```python
from build123d import *

# Parameters (mm, degrees)
BOSS_EXTRUDE1_DEPTH             = 12.7
BOSS_EXTRUDE4_REACH             = 14.7
BOSS_EXTRUDE4_DIRECTION_2_REACH = 14.7
SKETCH6_W                       = 16.51
SKETCH6_H                       = 15.748
CUT_EXTRUDE2_DEPTH              = 46.72
SKETCH11_W                      = 15.24
SKETCH11_H                      = 7.62
CUT_EXTRUDE3_DEPTH              = 3.81
SKETCH15_R                      = 3.2385
CUT_EXTRUDE4_DEPTH              = 25.4
SKETCH16_W                      = 6.35
SKETCH16_H                      = 21.59
BOSS_EXTRUDE5_DEPTH             = 15.24
SKETCH17_R                      = 0.635
CUT_EXTRUDE5_DEPTH              = 26.4


with BuildPart() as part:
    # Sketch1 → Boss-Extrude1 (new body, symmetric)
    with BuildSketch(Plane.XY):
        with BuildLine():
            Line((-15.24, 16.002), (-15.24, -25.4))
            Line((-15.24, -25.4), (15.24, -25.4))
            Line((15.24, -25.4), (15.24, 16.002))
            Line((15.24, 16.002), (2.794, 16.002))
            Line((2.794, 16.002), (2.794, 28.3845))
            Line((2.794, 28.3845), (6.477, 28.3845))
            ThreePointArc((6.477, 28.3845), (6.946330803, 28.698096816), (6.836210245, 29.251710245))
            Line((6.836210245, 29.251710245), (3.452459265, 32.635461224))
            ThreePointArc((3.452459265, 32.635461224), (2.628423959, 33.186064013), (1.656408041, 33.37941))
            Line((1.656408041, 33.37941), (-1.656408041, 33.37941))
            ThreePointArc((-1.656408041, 33.37941), (-2.628423959, 33.186064013), (-3.452459265, 32.635461224))
            Line((-3.452459265, 32.635461224), (-6.836210245, 29.251710245))
            ThreePointArc((-6.836210245, 29.251710245), (-6.946330803, 28.698096816), (-6.477, 28.3845))
            Line((-6.477, 28.3845), (-2.794, 28.3845))
            Line((-2.794, 28.3845), (-2.794, 16.002))
            Line((-2.794, 16.002), (-15.24, 16.002))
        make_face()
        Polygon((-4.106115114, 7.112), (-8.212230229, 0), (-4.106115114, -7.112), (4.106115114, -7.112), (8.212230229, 0), (4.106115114, 7.112), align=None, mode=Mode.SUBTRACT)
    extrude(amount=BOSS_EXTRUDE1_DEPTH, both=True)

    # Boss-Extrude4: up to this face of the body (flat: up to its plane)
    boss_extrude4_end = Plane(part.part.faces().sort_by_distance((-6.334610257, 28.951479763, 12.7))[0])
    # Sketch10 → Boss-Extrude4 (add, up to the picked face)
    with BuildSketch(Plane.XY, mode=Mode.PRIVATE) as boss_extrude4_sk1:
        Polygon((-15.24, -25.4), (-15.24, -46.99), (-30.48, -46.99), (-30.48, -50.8), (-11.43, -50.8), (-11.43, -25.4), align=None)
    boss_extrude4_tool1 = split(extrude(boss_extrude4_sk1.sketch, amount=BOSS_EXTRUDE4_REACH, mode=Mode.PRIVATE), bisect_by=boss_extrude4_end, keep=Keep.BOTH, mode=Mode.PRIVATE)
    add(boss_extrude4_tool1.solids().sort_by_distance((-14.9225, -36.195, 0))[0])

    # Boss-Extrude4 direction 2: up to this face of the body (flat: up to its plane)
    boss_extrude4_direction_2_end = Plane(part.part.faces().sort_by_distance((-6.334610257, 28.951479763, -12.7))[0])
    # Sketch10 → Boss-Extrude4 direction 2 (add, up to the picked face)
    with BuildSketch(Plane.XY, mode=Mode.PRIVATE) as boss_extrude4_direction_2_sk1:
        Polygon((-15.24, -25.4), (-15.24, -46.99), (-30.48, -46.99), (-30.48, -50.8), (-11.43, -50.8), (-11.43, -25.4), align=None)
    boss_extrude4_direction_2_tool1 = split(extrude(boss_extrude4_direction_2_sk1.sketch, amount=-BOSS_EXTRUDE4_DIRECTION_2_REACH, mode=Mode.PRIVATE), bisect_by=boss_extrude4_direction_2_end, keep=Keep.BOTH, mode=Mode.PRIVATE)
    add(boss_extrude4_direction_2_tool1.solids().sort_by_distance((-14.9225, -36.195, 0))[0])

    # Sketch6 → Cut-Extrude2 (cut, through all)
    with BuildSketch(Plane(origin=(15.24, 0, 0), x_dir=(0, 0, -1), z_dir=(1, 0, 0))):
        with Locations((0, -17.526)):
            Rectangle(SKETCH6_W, SKETCH6_H)
    extrude(amount=-CUT_EXTRUDE2_DEPTH, mode=Mode.SUBTRACT)

    # Sketch11 → Cut-Extrude3 (cut)
    with BuildSketch(Plane(origin=(0, -46.99, 0), x_dir=(1, 0, 0), z_dir=(0, 1, 0))):
        with Locations((-22.86, 0)):
            Rectangle(SKETCH11_W, SKETCH11_H)
    extrude(amount=-CUT_EXTRUDE3_DEPTH, mode=Mode.SUBTRACT)

    # Sketch15 → Cut-Extrude4 (cut)
    with BuildSketch(Plane.XY.offset(12.7)):
        with Locations((0, -19.05)):
            Circle(SKETCH15_R)
    extrude(amount=-CUT_EXTRUDE4_DEPTH, mode=Mode.SUBTRACT)

    # Sketch16 → Boss-Extrude5 (add)
    with BuildSketch(Plane.ZY.offset(15.24)):
        with Locations((9.525, -36.195)):
            Rectangle(SKETCH16_W, SKETCH16_H)
        with Locations((-9.525, -36.195)):
            Rectangle(SKETCH16_W, SKETCH16_H)
    extrude(amount=BOSS_EXTRUDE5_DEPTH)

    # Sketch17 → Cut-Extrude5 (cut, through all)
    with BuildSketch(Plane.XY.offset(12.7)):
        with Locations((-27.94, -31.75)):
            Circle(SKETCH17_R)
        with Locations((-27.94, -44.45)):
            Circle(SKETCH17_R)
    extrude(amount=-CUT_EXTRUDE5_DEPTH, mode=Mode.SUBTRACT)


solid = part.part
```
The model under review builds one solid part; all positions refer to its coordinate system, in mm. A direction names the side the tool comes from. Round coordinates to 2 decimals unless told otherwise and drop trailing zeros. Order: outer loops, then holes, each group sorted by start corner. A loop starts at its lowest first (then second) coordinate and runs counter-clockwise, first axis right, second up. Notation, with made-up numbers: (-22.5, -19) -> (32.5, -19) arc R23 ccw to (32.5, -3) -> close; hole circle Ø2 at (60.25, -23.75). An arc over 180 degrees is marked (long way). One line per item, written item: value. Start each with the question number.
Q1. Wall thickness on line 1 (Y direction, x = 0, z = -10.7); line 2 (Y direction, x = -27.94, z = -10) (3 decimals); line 3 (Z direction, x = -29, y = -44): over which ranges is each line inside the solid? List them lowest first.
Q2. Take a section at C-C (x = 0). Write out the cut boundary in (y, z) (1 decimal), and give its area (3 significant figures).
Q3. Take a section at B-B (y = -19.05). Write out the cut boundary in (x, z) (1 decimal).
Q4. Take a section at A-A (z = 5.5). Write out the cut boundary in (x, y).
Q5. Mouldability with a two-part tool opening along Z and no side actions: class faces 1 (the face through (-8, -19, -12.7)), 2 (the face through (4, -18, -8.255)), 3 (the face through (-30.48, -38, 9)) as released by +Z, released by -Z, zero draft, split by the parting line, or undercut.
Q6. Machinability: for faces 4 (the face through (-23, -49, -3.81)), 5 (the face through (0, 7.112, 0)), 6 (the face through (2, -25.4, 11)), 7 (the face through (-5, 28.384, 0)), which of the approach directions +Z, -Z, +X, -X, +Y, -Y give a long, thin tool a straight path to every point of the face, cutting with its end or side? Answer none if there is none.
Q7. Clearance check with flat-ended pins moving along their axes: pin 1 Ø2 at (x, y) = (-27.94, -44.45) entering from +Z; pin 2 Ø10 at (x, z) = (-23, -6.5) entering from +Y; pin 3 Ø4 at (x, z) = (-9.5, 1.5) entering from +Y; pin 4 Ø1.8 at (x, z) = (5, -2) entering from -Y. State where each tip first meets the part, or that it passes through.
Q8. Take a section at D-D (y = -40). Write out the cut boundary in (x, z), and give its area (3 significant figures).
Reported:
1. line 1: y = -25.4 to -22.29, -15.81 to -7.11, 7.11 to 33.38
1. line 2: y = -50.8 to -45.085, -43.815 to -32.385, -31.115 to -25.4
1. line 3: z = -12.7 to -6.35, 6.35 to 12.7
2. outline: (-25.4, -12.7) -> (-22.3, -12.7) -> (-22.3, -8.3) -> (-25.4, -8.3) -> close; (-25.4, 8.3) -> (-22.3, 8.3) -> (-22.3, 12.7) -> (-25.4, 12.7) -> close; (-15.8, -12.7) -> (-7.1, -12.7) -> (-7.1, 12.7) -> (-15.8, 12.7) -> (-15.8, 8.3) -> (-9.7, 8.3) -> (-9.7, -8.3) -> (-15.8, -8.3) -> close; (7.1, -12.7) -> (33.4, -12.7) -> (33.4, 12.7) -> (7.1, 12.7) -> close
2. area: 814 mm2
3. outline: (-15.2, -12.7) -> (-3.2, -12.7) -> (-3.2, -8.3) -> (-15.2, -8.3) -> close; (-15.2, 8.3) -> (-3.2, 8.3) -> (-3.2, 12.7) -> (-15.2, 12.7) -> close; (3.2, -12.7) -> (15.2, -12.7) -> (15.2, -8.3) -> (3.2, -8.3) -> close; (3.2, 8.3) -> (15.2, 8.3) -> (15.2, 12.7) -> (3.2, 12.7) -> close
4. outline: (-30.48, -50.8) -> (-11.43, -50.8) -> (-11.43, -25.4) -> (-15.24, -25.4) -> (-15.24, -46.99) -> (-30.48, -46.99) -> close; (-15.24, -9.65) -> (15.24, -9.65) -> (15.24, 16) -> (2.79, 16) -> (2.79, 28.38) -> (6.48, 28.38) arc R0.51 ccw to (6.84, 29.25) -> (3.45, 32.64) arc R2.54 ccw to (1.66, 33.38) -> (-1.66, 33.38) arc R2.54 ccw to (-3.45, 32.64) -> (-6.84, 29.25) arc R0.51 ccw to (-6.48, 28.38) -> (-2.79, 28.38) -> (-2.79, 16) -> (-15.24, 16) -> close; hole (-8.21, 0) -> (-4.11, -7.11) -> (4.11, -7.11) -> (8.21, 0) -> (4.11, 7.11) -> (-4.11, 7.11) -> close
5. face 1: released by -Z
5. face 2: undercut
5. face 3: zero draft
6. face 4: -X, +Y, -Y
6. face 5: +Z, -Z
6. face 6: +Z, -Z, +X, -Y
6. face 7: +Z, -Z, -X
7. pin 1: stops at z = 12.7
7. pin 2: stops at y = -25.4
7. pin 3: stops at y = 16
7. pin 4: stops at y = -9.65
8. outline: (-30.48, -12.7) -> (-11.43, -12.7) -> (-11.43, 12.7) -> (-30.48, 12.7) -> (-30.48, 6.35) -> (-15.24, 6.35) -> (-15.24, -6.35) -> (-30.48, -6.35) -> close
8. area: 290 mm2
